```python
from build123d import *
from build123d.topology import SkipClean

# Parameters (mm, degrees)
SKETCH1_R           = 9.375
END_CAP_MAIN_DEPTH  = 13.65
FILLET1_R           = 1.4
SKETCH2_R           = 4.4
END_CAP_CUT_DEPTH   = 9.3
FILLET2_R           = 1
SKETCH16_R          = 8.105
CUT_EXTRUDE12_DEPTH = 2.5
SKETCH5_3_R         = 8.105
BOSS_EXTRUDE4_DEPTH = 2.5
SKETCH4_R           = 6.9
SKETCH5_R           = 8.105
SKETCH6_W           = 2.4
SKETCH6_H           = 13.3
BOSS_EXTRUDE2_DEPTH = 20.72
CUT_EXTRUDE2_REACH  = 153.053
CUT_EXTRUDE4_DEPTH  = 0.655
CUT_EXTRUDE9_REACH  = 153.052
CUT_EXTRUDE10_REACH = 153.052
BOSS_EXTRUDE3_DEPTH = 2.4
CUT_EXTRUDE11_REACH = 153.052
SKETCH15_R          = 2.2


with BuildPart() as part:
    # Sketch1 → End Cap Main (new body)
    with BuildSketch(Plane.XY):
        Circle(SKETCH1_R)
    extrude(amount=END_CAP_MAIN_DEPTH)

    # Fillet1
    fillet1_edges = [part.edges().sort_by_distance(p)[0] for p in [
        (-9.375, 0, 0),
    ]]
    fillet(fillet1_edges, radius=FILLET1_R)

    # Sketch2 → End Cap cut (cut)
    with BuildSketch(Plane(origin=(0, 0, 0), x_dir=(-1, 0, 0), z_dir=(0, 0, -1))):
        Circle(SKETCH2_R)
    extrude(amount=-END_CAP_CUT_DEPTH, mode=Mode.SUBTRACT)

    # Fillet2
    fillet2_edges = [part.edges().sort_by_distance(p)[0] for p in [
        (4.4, 0, 0),
    ]]
    fillet(fillet2_edges, radius=FILLET2_R)

    # Sketch16 → Cut-Extrude12 (cut)
    with BuildSketch(Plane.XY.offset(13.65)):
        Circle(SKETCH16_R)
    extrude(amount=-CUT_EXTRUDE12_DEPTH, mode=Mode.SUBTRACT)

    # Sketch5<3> → Boss-Extrude4 (add)
    with BuildSketch(Plane.XY.offset(13.65)):
        Circle(SKETCH5_3_R)
    extrude(amount=-BOSS_EXTRUDE4_DEPTH)

    # Sketch4 → Loft1 section 0
    with BuildSketch(Plane.XY.offset(129.67)):
        Circle(SKETCH4_R)
    # Sketch5 → Loft1 section 1
    with BuildSketch(Plane.XY.offset(13.65)):
        Circle(SKETCH5_R)
    loft()

    # Sketch6 → Boss-Extrude2 (add)
    with BuildSketch(Plane.XY.offset(129.67)):
        Rectangle(SKETCH6_W, SKETCH6_H)
    extrude(amount=BOSS_EXTRUDE2_DEPTH)

    # Sketch9 → Cut-Extrude2 (cut, up to next)
    with BuildSketch(Plane(origin=(1.2, 0, 0), x_dir=(0, 0, -1), z_dir=(1, 0, 0)), mode=Mode.PRIVATE) as cut_extrude2_sk1:
        with BuildLine():
            Line((-150.39, 6.65), (-150.39, -6.65))
            Line((-150.39, -6.65), (-143.73925134, -6.65))
            ThreePointArc((-143.73925134, -6.65), (-150.38925134, 0), (-143.73925134, 6.65))
            Line((-143.73925134, 6.65), (-150.39, 6.65))
        make_face()
    cut_extrude2_tool1 = extrude(cut_extrude2_sk1.sketch, amount=-CUT_EXTRUDE2_REACH, mode=Mode.PRIVATE) & part.part
    add(cut_extrude2_tool1.solids().sort_by_distance((1.2, 6.501298, 147.064626))[0], mode=Mode.SUBTRACT)

    # Sketch10 → Cut-Extrude4 (cut)
    with SkipClean():  # the faces are left unmerged after this step: merging them gives an invalid solid
        with BuildSketch(Plane(origin=(1.2, 0, 0), x_dir=(0, 0, -1), z_dir=(1, 0, 0))):
            with BuildLine():
                Line((-143.73925134, 6.65), (-133.16425134, 6.65))
                ThreePointArc((-133.16425134, 6.65), (-136.114103218, 5.959939085), (-138.45175134, 4.032969594))
                ThreePointArc((-138.45175134, 4.032969594), (-140.789399463, 5.959939085), (-143.73925134, 6.65))
            make_face()
        cut_extrude4 = extrude(amount=-CUT_EXTRUDE4_DEPTH, mode=Mode.SUBTRACT)

    # Mirror1: Cut-Extrude4 across plane
    with SkipClean():  # the faces are left unmerged after this step: merging them gives an invalid solid
        add(cut_extrude4.mirror(Plane(origin=(0, 0, 0), x_dir=(0, 0, 1), z_dir=(1, 0, 0))), mode=Mode.SUBTRACT)

    # Sketch12 → Cut-Extrude9 (cut, up to next)
    with BuildSketch(Plane(origin=(1.2, 0, 0), x_dir=(0, 0, -1), z_dir=(1, 0, 0)), mode=Mode.PRIVATE) as cut_extrude9_sk1:
        with BuildLine():
            Line((-143.73925134, -3.925), (-143.73925134, -6.65))
            Line((-143.73925134, -6.65), (-139.81425134, -6.65))
            Line((-139.81425134, -6.65), (-139.81425134, 0))
            ThreePointArc((-139.81425134, 0), (-146.514645456, 2.775394116), (-143.73925134, -3.925))
        make_face()
    cut_extrude9_tool1 = extrude(cut_extrude9_sk1.sketch, amount=-CUT_EXTRUDE9_REACH, mode=Mode.PRIVATE) & part.part
    add(cut_extrude9_tool1.solids().sort_by_distance((1.2, -1.067806, 143.241366))[0], mode=Mode.SUBTRACT)

    # Sketch13 → Cut-Extrude10 (cut, up to next)
    with BuildSketch(Plane(origin=(1.2, 0, 0), x_dir=(0, 0, -1), z_dir=(1, 0, 0)), mode=Mode.PRIVATE) as cut_extrude10_sk1:
        with BuildLine():
            Line((-139.81425134, 0), (-139.81425134, -6.65))
            Line((-139.81425134, -6.65), (-133.16425134, -6.65))
            ThreePointArc((-133.16425134, -6.65), (-137.866511435, -4.702260095), (-139.81425134, 0))
        make_face()
    cut_extrude10_tool1 = extrude(cut_extrude10_sk1.sketch, amount=-CUT_EXTRUDE10_REACH, mode=Mode.PRIVATE) & part.part
    add(cut_extrude10_tool1.solids().sort_by_distance((1.2, -5.164603, 138.328855))[0], mode=Mode.SUBTRACT)

    # Sketch14 → Boss-Extrude3 (add)
    with SkipClean():  # the faces are left unmerged after this step: merging them gives an invalid solid
        with BuildSketch(Plane(origin=(1.2, 0, 0), x_dir=(0, 0, -1), z_dir=(1, 0, 0))):
            with BuildLine():
                Line((-143.73925134, -3.925), (-143.73925134, -6.65))
                ThreePointArc((-143.73925134, -6.65), (-142.37675134, -5.2875), (-143.73925134, -3.925))
            make_face()
        extrude(amount=-BOSS_EXTRUDE3_DEPTH)

    # Sketch15 → Cut-Extrude11 (cut, up to next)
    with BuildSketch(Plane(origin=(1.2, 0, 0), x_dir=(0, 0, -1), z_dir=(1, 0, 0)), mode=Mode.PRIVATE) as cut_extrude11_sk1:
        with Locations((-133.16425134, 0)):
            Circle(SKETCH15_R)
    cut_extrude11_tool1 = extrude(cut_extrude11_sk1.sketch, amount=-CUT_EXTRUDE11_REACH, mode=Mode.PRIVATE) & part.part
    add(cut_extrude11_tool1.solids().sort_by_distance((1.2, 0, 133.164251))[0], mode=Mode.SUBTRACT)


solid = part.part
```
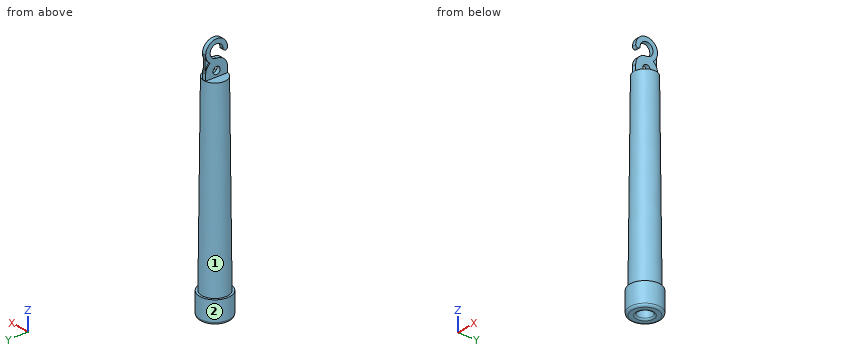
The model under review builds one solid part; all positions refer to its coordinate system, in mm. Face numbers are marked on the shaded views. A direction names the side the tool comes from. Give positions to 0.01 mm unless a question says otherwise; leave off trailing zeros. Write each loop counter-clockwise with the first axis right and the second up, starting at its lowest first coordinate (ties: lowest second). Pieces come first, ordered by that corner, then holes. Notation, with made-up numbers: M 17.25,20 L 25.25,20 A17 ccw 25.25,51 Z; hole C 32,70 d9. An arc over 180 degrees is marked long. Write each question's results on one line, items separated by ' | '. Start each with the question number.
1. We need section A-A (z = 23). Write out the cut boundary in (x, y), and give its area (3 significant figures).
2. We need section B-B (z = 58.5). Write out the cut boundary in (x, y), and give its area (3 significant figures).
3. For the marked faces 1 and 2, list the 3-axis set-ups (+Z, -Z, +X, -X, +Y, -Y) from which the entire face can be reached by the end or side of a thin tool; tool diameter is ignored.
4. Insertion check: pin 1 Ø3 at (x, y) = (5, -3.5) entering from +Z; pin 2 Ø6.5 at (y, z) = (0, 143.74) entering from -X; pin 3 Ø1 at (y, z) = (-7.5, 40.5) entering from -X; pin 4 Ø2.5 at (x, z) = (0.5, 137.5) entering from +Y. Each pin has a flat end and moves straight along its axis. Give the tip position at first contact, or say it passes through.
5. For probe 1 along Z at (x, y) = (-0.25, -2); probe 2 along Z at (x, y) = (-5.5, -3.5); probe 3 along Z at (x, y) = (-1.5, -3.5), list the stretches that pass through material, from the lowest coordinate up. Write a range as [from, to].
Results found:
1) outline: C 0,0 d16.02 | area: 201 mm^2
2) outline: C 0,0 d15.28 | area: 183 mm^2
3) face 1: +Z | face 2: +Z, -Z
4) pin 1: stops at z = 129.67 | pin 2: passes through | pin 3: stops at x = -3.5 | pin 4: stops at y = 6.65
5) probe 1: z = [9.3, 132.25], [134.08, 139.51], [147.12, 150.08] | probe 2: z = [0, 129.67] | probe 3: z = [9.3, 129.67]
